Check sheet for the modelled part. Datum: model origin and axes. Units: mm. Face numbers are marked on the shaded views. A direction names the side the tool comes from. Coordinates: 2 decimals unless noted, no trailing zeros. Order: outer loops, then holes, each group sorted by start corner. A loop starts at its lowest first (then second) coordinate and runs counter-clockwise, first axis right, second up.
1. Set-up check for the marked faces 1 and 2: record each of +Z, -Z, +X, -X, +Y, -Y from which the full face is reachable in a straight line by a thin tool's end or side.
2. Cross-section at A-A (x = 121.5). Enter the section's corners in (y, z).
3. Gauge pin test, flat ends, axial feed: pin 1 Ø6.5 at (x, y) = (50, 30) entering from -Z; pin 2 Ø8 at (x, y) = (146.5, 11) entering from +Z; pin 3 Ø1 at (x, z) = (405, -23.5) entering from +Y; pin 4 Ø3 at (x, y) = (230, 3) entering from +Z. Record the tip position at first contact, or that the pin passes through.
4. Cross-section at C-C (z = -5). Enter the section's corners in (x, y).
5. Thickness scan on line 1 (X direction, y = 30, z = -39.4); line 2 (Z direction, x = 266.5, y = 19.5); line 3 (Y direction, x = 69.5, z = -25.5). Record the ranges inside material, lowest first.
6. Cross-section at B-B (y = 7). Enter the section's corners in (x, z), then the cut area to 3 significant figures.
```python
from build123d import *

# Parameters (mm, degrees)
SKETCH_1_W                       = 480
SKETCH_1_H                       = 40
SM_BASE_FLANGE_1_DEPTH           = 2
SM_EDGE_FLANGE_1_STRIP_W         = 12
SM_EDGE_FLANGE_1_STRIP_H         = 2
SM_EDGE_FLANGE_1_STRIP_CUT_DEPTH = 480
SM_EDGE_FLANGE_1_DEPTH           = 480
SKETCH_9_R                       = 2.5
CUT_EXTRUDE_1_DEPTH              = 484.160428843


# Sheet-metal steps are written as plain solids
with BuildPart() as part:
    # Sketch 1 → Базовая кромка1 (new body)
    with BuildSketch(Plane(origin=(0, 0, 0), x_dir=(1, 0, 0), z_dir=(0, 1, 0))):
        with Locations((240, 20)):
            Rectangle(SKETCH_1_W, SKETCH_1_H)
    extrude(amount=-SM_BASE_FLANGE_1_DEPTH)

    # Ребро-кромка1 strip (across the edge) → Ребро-кромка1 strip cut (cut)
    with BuildSketch(Plane(origin=(480, 0, -40), x_dir=(0, 0, 1), z_dir=(-1, 0, 0))):
        with Locations((-2, -1)):
            Rectangle(SM_EDGE_FLANGE_1_STRIP_W, SM_EDGE_FLANGE_1_STRIP_H)
    extrude(amount=SM_EDGE_FLANGE_1_STRIP_CUT_DEPTH, mode=Mode.SUBTRACT)

    # Ребро-кромка1 section (across the edge) → Ребро-кромка1 (add)
    with BuildSketch(Plane(origin=(480, 0, -40), x_dir=(0, 0, 1), z_dir=(-1, 0, 0))):
        with BuildLine():
            Line((0, 2), (0, 38))
            Line((0, 38), (2, 38))
            Line((2, 38), (2, 2))
            ThreePointArc((2, 2), (2.585786438, 0.585786438), (4, 0))
            Line((4, 0), (4, -2))
            ThreePointArc((4, -2), (1.171572875, -0.828427125), (0, 2))
        make_face()
    extrude(amount=SM_EDGE_FLANGE_1_DEPTH)

    # Эскиз9 → Вырез-Вытянуть1 (cut, through all)
    with BuildSketch(Plane(origin=(0, 0, -40), x_dir=(-1, 0, 0), z_dir=(0, 0, -1))):
        with Locations(Location((-450, 30, 0), (0, 0, 90))):
            Circle(SKETCH_9_R)
        with Locations(Location((-350, 30, 0), (0, 0, 90))):
            Circle(SKETCH_9_R)
        with Locations(Location((-250, 30, 0), (0, 0, 90))):
            Circle(SKETCH_9_R)
        with Locations(Location((-150, 30, 0), (0, 0, 90))):
            Circle(SKETCH_9_R)
        with Locations(Location((-50, 30, 0), (0, 0, 90))):
            Circle(SKETCH_9_R)
    extrude(amount=-CUT_EXTRUDE_1_DEPTH, mode=Mode.SUBTRACT)


solid = part.part
```
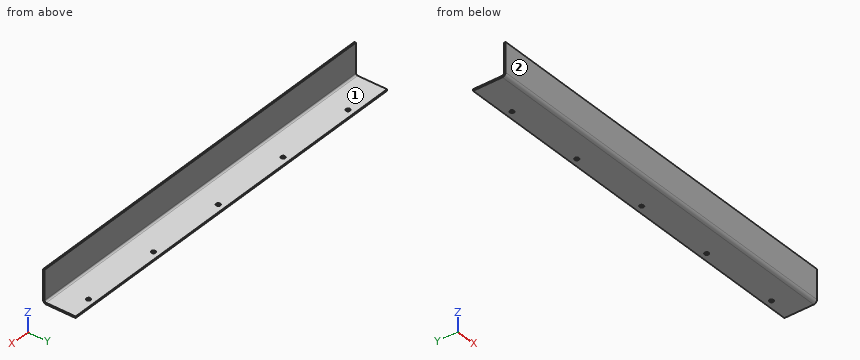
Data:
1. face 1: +Z, +X, -X, +Y
1. face 2: +Z, -Z, +X, -X, -Y
2. outline: (-2, -36) arc R4 ccw to (2, -40) - (38, -40) - (38, -38) - (2, -38) arc R2 cw to (0, -36) - (0, 0) - (-2, 0) - close
3. pin 1: stops at z = -40
3. pin 2: stops at z = -38
3. pin 3: stops at y = 0
3. pin 4: stops at z = -37.94
4. outline: (0, -2) - (480, -2) - (480, 0) - (0, 0) - close
5. line 1: x = 0 to 47.5, 52.5 to 147.5, 152.5 to 247.5, 252.5 to 347.5, 352.5 to 447.5, 452.5 to 480
5. line 2: z = -40 to -38
5. line 3: y = -2 to 0
6. outline: (0, -40) - (480, -40) - (480, -38) - (0, -38) - close
6. area: 960 mm2
